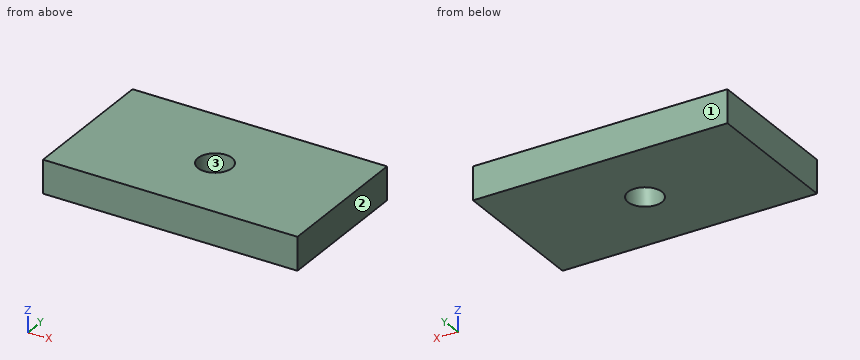
from build123d import *

# Parameters (mm, degrees)
ESQUISSE1_W                  = 30
ESQUISSE1_H                  = 17
BOSS_EXTRU_1_DEPTH           = 3.9
F_4_0_4_DIAMETER_HOLE1_D     = 4
F_4_0_4_DIAMETER_HOLE1_DEPTH = 3.9


with BuildPart() as part:
    # Esquisse1 → Boss.-Extru.1 (new body)
    with BuildSketch(Plane.XY):
        with Locations((0, 8.5)):
            Rectangle(ESQUISSE1_W, ESQUISSE1_H)
    extrude(amount=BOSS_EXTRU_1_DEPTH)

    # Ø4.0 (4) Diameter Hole1
    with Locations(Plane(origin=(0, 0, 0), x_dir=(-1, 0, 0), z_dir=(0, 0, -1))):
        with Locations((0, 8.5)):
            Hole(F_4_0_4_DIAMETER_HOLE1_D / 2, depth=F_4_0_4_DIAMETER_HOLE1_DEPTH)


solid = part.part
Here's how the part is built. I have some questions about the finished solid (model axes, mm). Face numbers are marked on the shaded views. Give positions to 0.01 mm unless a question says otherwise; leave off trailing zeros. Order: outer loops, then holes, each group sorted by start corner. A loop starts at its lowest first (then second) coordinate and runs counter-clockwise, first axis right, second up. Notation, with made-up numbers: (32, -38.75) -> (41, -38.75) arc R19 cw to (41, -23.75) -> close; hole circle Ø2 at (72.5, 3). An arc over 180 degrees is marked (long way). Use a Markdown table: item, result. Add a question column.
Item 1: Imagine slicing it at C-C on y = 7.5. Please give me the cut outline in (x, z), plus the area to 3 significant figures.
Item 2: Imagine slicing it at B-B on z = 1.1. Please give me the cut outline in (x, y), plus the area to 3 significant figures.
Item 3: Imagine slicing it at A-A on x = 0. Please give me the cut outline in (y, z).
Item 4: If we mould it in two halves opening along X, with no side actions, what happens to the marked faces 1, 2 and 3? For each: pulls with the +X half, pulls with the -X half, needs draft (parallel to the pull), parting line crosses it, or undercut.
Item 5: I need wall thicknesses on line 1 (Y direction, x = 0, z = 2.95); line 2 (X direction, y = 9.5, z = 1.95). Which ranges of each line are inside material? Lowest first, please.
Data:
| question | item | result |
|---|---|---|
| 1 | outline | (-15, 0) -> (-1.73, 0) -> (-1.73, 3.9) -> (-15, 3.9) -> close; (1.73, 0) -> (15, 0) -> (15, 3.9) -> (1.73, 3.9) -> close |
| 1 | area | 103 mm² |
| 2 | outline | (-15, 0) -> (15, 0) -> (15, 17) -> (-15, 17) -> close; hole circle Ø4 at (0, 8.5) |
| 2 | area | 497 mm² |
| 3 | outline | (0, 0) -> (6.5, 0) -> (6.5, 3.9) -> (0, 3.9) -> close; (10.5, 0) -> (17, 0) -> (17, 3.9) -> (10.5, 3.9) -> close |
| 4 | face 1 | needs draft |
| 4 | face 2 | pulls with the +X half |
| 4 | face 3 | undercut |
| 5 | line 1 | y = 0 to 6.5, 10.5 to 17 |
| 5 | line 2 | x = -15 to -1.73, 1.73 to 15 |
